Source: CAD feature listing. Evaluate the final solid. Frame: model axes, mm. A direction names the side the tool comes from. Coordinates: 2 decimals unless noted, no trailing zeros. Order: outer loops, then holes, each group sorted by start corner. A loop starts at its lowest first (then second) coordinate and runs counter-clockwise, first axis right, second up.
```python
from build123d import *

# Parameters (mm, degrees)
F1_DEPTH = 6.35
F2_R     = 12.7
F2_R_2   = 9.525
F2_R_3   = 3.175
F3_DEPTH = 1.5875
F4_W     = 3.175
F4_H     = 25.4
F5_DEPTH = 3.175
F6_W     = 38.1
F6_H     = 25.4
F7_DEPTH = 3.175


with BuildPart() as f1:
    # F0 (on Top) → F1 (new body)
    with BuildSketch(Plane.XY):
        Polygon((-15.875, 0), (-60.325, 0), (-76.2, -15.875), (-76.2, -60.325), (-60.325, -76.2), (-15.875, -76.2), (0, -60.325), (0, -15.875), align=None)
    extrude(amount=F1_DEPTH)

    # F2 (on face) → F3 (join)
    with BuildSketch(Plane.XY.offset(6.35)):
        Polygon((0, -15.875), (-15.875, 0), (-60.325, 0), (-76.2, -15.875), (-76.2, -60.325), (-60.325, -76.2), (-15.875, -76.2), (0, -60.325), align=None)
        Polygon((-3.175, -17.190128), (-3.175, -59.009872), (-17.190128, -73.025), (-59.009872, -73.025), (-73.025, -59.009872), (-73.025, -17.190128), (-59.009872, -3.175), (-17.190128, -3.175), align=None, mode=Mode.SUBTRACT)
        with BuildLine():
            Line((-38.1, -66.675), (-33.609872, -62.184872))
            ThreePointArc((-33.609872, -62.184872), (-14.015128, -62.184872), (-14.015128, -42.590128))
            Line((-14.015128, -42.590128), (-9.525, -38.1))
            Line((-9.525, -38.1), (-14.015128, -33.609872))
            ThreePointArc((-14.015128, -33.609872), (-14.015128, -14.015128), (-33.609872, -14.015128))
            Line((-33.609872, -14.015128), (-38.1, -9.525))
            Line((-38.1, -9.525), (-42.590128, -14.015128))
            ThreePointArc((-42.590128, -14.015128), (-62.184872, -14.015128), (-62.184872, -33.609872))
            Line((-62.184872, -33.609872), (-66.675, -38.1))
            Line((-66.675, -38.1), (-62.184872, -42.590128))
            ThreePointArc((-62.184872, -42.590128), (-62.184872, -62.184872), (-42.590128, -62.184872))
            Line((-42.590128, -62.184872), (-38.1, -66.675))
        make_face()
        with BuildLine():
            ThreePointArc((-33.268461, -18.846667), (-16.260192, -16.260192), (-18.846667, -33.268461))
            Line((-18.846667, -33.268461), (-14.015128, -38.1))
            Line((-14.015128, -38.1), (-18.846667, -42.931539))
            ThreePointArc((-18.846667, -42.931539), (-16.260192, -59.939808), (-33.268461, -57.353333))
            Line((-33.268461, -57.353333), (-38.1, -62.184872))
            Line((-38.1, -62.184872), (-42.931539, -57.353333))
            ThreePointArc((-42.931539, -57.353333), (-59.939808, -59.939808), (-57.353333, -42.931539))
            Line((-57.353333, -42.931539), (-62.184872, -38.1))
            Line((-62.184872, -38.1), (-57.353333, -33.268461))
            ThreePointArc((-57.353333, -33.268461), (-59.939808, -16.260192), (-42.931539, -18.846667))
            Line((-42.931539, -18.846667), (-38.1, -14.015128))
            Line((-38.1, -14.015128), (-33.268461, -18.846667))
        make_face(mode=Mode.SUBTRACT)
        with Locations((-38.1, -38.1)):
            Circle(F2_R)
        with Locations((-38.1, -38.1)):
            Circle(F2_R_2, mode=Mode.SUBTRACT)
        with Locations((-52.3875, -52.3875)):
            Circle(F2_R_3)
        with Locations((-23.8125, -52.3875)):
            Circle(F2_R_3)
        with Locations((-23.8125, -23.8125)):
            Circle(F2_R_3)
        with Locations((-52.3875, -23.8125)):
            Circle(F2_R_3)
    extrude(amount=F3_DEPTH)

    # F4 (on face) → F5 (join)
    with BuildSketch(Plane(origin=(0, 0, 0), x_dir=(1, 0, 0), z_dir=(0, 0, -1))):
        with Locations((-55.5625, 38.1)):
            Rectangle(F4_W, F4_H)
        with Locations((-20.6375, 38.1)):
            Rectangle(F4_W, F4_H)
    extrude(amount=F5_DEPTH)

    # F6 (on face) → F7 (join)
    with BuildSketch(Plane(origin=(0, 0, -3.175), x_dir=(1, 0, 0), z_dir=(0, 0, -1))):
        with Locations((-38.1, 38.1)):
            Rectangle(F6_W, F6_H)
    extrude(amount=F7_DEPTH)


solid = f1.part
```
Q1. Pin query (flat end, axial travel): P1, Ø7, axis at y = -34, z = -4.5, coming from the -X side; P2, Ø8, axis at x = -11.5, z = 6, coming from the -Y side (3 decimals); P3, Ø1, axis at y = -35, z = -2, coming from the +X side. Return the tip coordinate at first contact, or that it passes through.
Solutions:
P1: stops at x = -57.15
P2: stops at y = -75.825
P3: stops at x = -19.05
Q2. Section query A-A on z = 2.25. Output: boundary loops of the cut face in (x, y) (3 decimals).
Solutions:
outline: (-76.2, -60.325) - (-60.325, -76.2) - (-15.875, -76.2) - (0, -60.325) - (0, -15.875) - (-15.875, 0) - (-60.325, 0) - (-76.2, -15.875) - close
Q3. Pull-direction query (X, two-part tool) for faces 1 (the flat face through (-38, -25.4, -5)), 2 (the cylindrical face through (-60.135, -16.461, 7.133)), 3 (the flat face through (-68.151, -7.826, 3.913)), 4 (the cylindrical face through (-49.455, -25.029, 7.133)); classes: pulls with the +X half, pulls with the -X half, needs draft (parallel to the pull), parting line crosses it, or undercut.
Solutions:
face 1: needs draft
face 2: undercut
face 3: pulls with the -X half
face 4: undercut
Q4. Material intervals for line 1 along Y through (x, z) = (-38.1, 7.2) (3 decimals); line 2 along Z through (x, y) = (-24, -43.5) (3 decimals); line 3 along X through (y, z) = (-16, 7.5), sorted ascending.
Solutions:
line 1: y = -76.2 to -73.025, -66.675 to -62.185, -50.8 to -47.625, -28.575 to -25.4, -14.015 to -9.525, -3.175 to 0
line 2: z = -6.35 to -3.175, 0 to 6.35
line 3: x = -76.2 to -71.83, -63.83 to -59.67, -45.1 to -40.08, -36.12 to -31.1, -16.53 to -12.37, -4.37 to 0
Q5. Set-up query: faces 5 (the flat face through (-35.824, -11.801, 7.133)), 6 (the flat face through (-38, -76.2, 4)), 7 (the flat face through (-38, -38, -3.175)). Return all of +Z, -Z, +X, -X, +Y, -Y with unobstructed straight access to the full face (end or side cutting, diameter ignored); none if empty.
Solutions:
face 5: +Z
face 6: +Z, -Z, +X, -X, -Y
face 7: +Y, -Y
